Check sheet for the modelled part. Datum: model origin and axes. Units: mm. Face numbers are marked on the shaded views. A direction names the side the tool comes from. Give positions to 0.01 mm unless a question says otherwise; leave off trailing zeros. Order: outer loops, then holes, each group sorted by start corner. A loop starts at its lowest first (then second) coordinate and runs counter-clockwise, first axis right, second up.
from build123d import *

# Parameters (mm, degrees)
SKETCH1_R               = 5
BOSS_EXTRUDE1_DEPTH     = 40
SKETCH2_R               = 9
BOSS_EXTRUDE2_DEPTH     = 10
SKETCH3_R               = 5
BOSS_EXTRUDE3_DEPTH     = 10
BOSS_EXTRUDE4_DEPTH     = 20
SKETCH6_R               = 5
BOSS_EXTRUDE5_DEPTH     = 8
SKETCH5_W               = 30
SKETCH5_H               = 5.5
CUT_EXTRUDE1_DEPTH      = 10
CUT_EXTRUDE1_DEPTH_BACK = 10
SKETCH8_R               = 1.5
CUT_EXTRUDE2_DEPTH      = 2


with BuildPart() as part:
    # Sketch1 → Boss-Extrude1 (new body)
    with BuildSketch(Plane.XY):
        Circle(SKETCH1_R)
    extrude(amount=BOSS_EXTRUDE1_DEPTH)

    # Sketch2 → Boss-Extrude2 (add)
    with BuildSketch(Plane(origin=(0, 0, 0), x_dir=(-1, 0, 0), z_dir=(0, 0, -1))):
        Circle(SKETCH2_R)
    extrude(amount=BOSS_EXTRUDE2_DEPTH)

    # Sketch3 → Boss-Extrude3 (add)
    with BuildSketch(Plane(origin=(0, 0, -10), x_dir=(-1, 0, 0), z_dir=(0, 0, -1))):
        Circle(SKETCH3_R)
    extrude(amount=BOSS_EXTRUDE3_DEPTH)

    # Sketch4 → Boss-Extrude4 (add)
    with BuildSketch(Plane(origin=(0, 0, -20), x_dir=(-1, 0, 0), z_dir=(0, 0, -1))):
        Polygon((-5, 0), (-2.5, -4.330127019), (2.5, -4.330127019), (5, 0), (2.5, 4.330127019), (-2.5, 4.330127019), align=None)
    extrude(amount=BOSS_EXTRUDE4_DEPTH)

    # Sketch6 → Boss-Extrude5 (add)
    with BuildSketch(Plane.XY.offset(40)):
        Circle(SKETCH6_R)
    extrude(amount=BOSS_EXTRUDE5_DEPTH)

    # Sketch5 → Cut-Extrude1 (cut, two sides)
    with BuildSketch(Plane(origin=(0, 0, 0), x_dir=(0, 0, -1), z_dir=(1, 0, 0))) as cut_extrude1_sk:
        with Locations((-30, 2.25)):
            Rectangle(SKETCH5_W, SKETCH5_H)
    extrude(amount=CUT_EXTRUDE1_DEPTH, mode=Mode.SUBTRACT)
    extrude(cut_extrude1_sk.sketch, amount=-CUT_EXTRUDE1_DEPTH_BACK, mode=Mode.SUBTRACT)

    # Sketch8 → Cut-Extrude2 (cut)
    with BuildSketch(Plane(origin=(0, -0.5, 0), x_dir=(1, 0, 0), z_dir=(0, 1, 0))):
        with Locations((0, -40)):
            Circle(SKETCH8_R)
        with Locations((0, -20)):
            Circle(SKETCH8_R)
    extrude(amount=-CUT_EXTRUDE2_DEPTH, mode=Mode.SUBTRACT)


solid = part.part
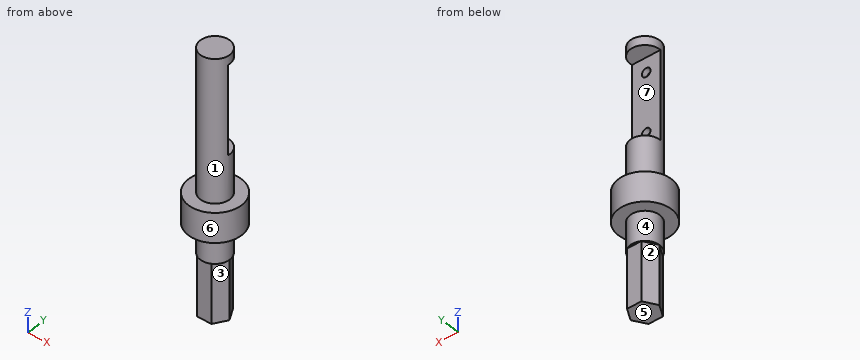
1) Draft check along Z on the marked faces 5, 6 and 7. Enter one of: +Z half, -Z half, draft (parallel to the pull), parting line (faces both ways), or undercut.
Recorded:
face 5: -Z half
face 6: draft
face 7: undercut
2) Set-up check for the marked faces 1, 2, 3 and 4: record each of +Z, -Z, +X, -X, +Y, -Y from which the full face is reachable in a straight line by a thin tool's end or side.
Recorded:
face 1: +Z
face 2: -Z, -X, +Y
face 3: -Z, +X, -Y
face 4: -Z
3) Section check B-B, the plane y = 2.25. Record the cut outline in (x, z), then the cut area to 3 significant figures.
Recorded:
outline: (-8.71, -10) - (-4.47, -10) - (-4.47, -20) - (-3.7, -20) - (-3.7, -40) - (3.7, -40) - (3.7, -20) - (4.47, -20) - (4.47, -10) - (8.71, -10) - (8.71, 0) - (4.47, 0) - (4.47, 15) - (-4.47, 15) - (-4.47, 0) - (-8.71, 0) - close; (-4.47, 45) - (4.47, 45) - (4.47, 48) - (-4.47, 48) - close
area: 572 mm2
4) Section check A-A, the plane x = 0. Record the cut outline in (y, z), then the cut area to 3 significant figures.
Recorded:
outline: (-9, -10) - (-5, -10) - (-5, -20) - (-4.33, -20) - (-4.33, -40) - (4.33, -40) - (4.33, -20) - (5, -20) - (5, -10) - (9, -10) - (9, 0) - (5, 0) - (5, 15) - (-0.5, 15) - (-0.5, 18.5) - (-2.5, 18.5) - (-2.5, 21.5) - (-0.5, 21.5) - (-0.5, 38.5) - (-2.5, 38.5) - (-2.5, 41.5) - (-0.5, 41.5) - (-0.5, 45) - (5, 45) - (5, 48) - (-5, 48) - (-5, 0) - (-9, 0) - close
area: 756 mm2
5) Section check C-C, the plane z = -28.5. Record the cut outline in (x, y).
Recorded:
outline: (-5, 0) - (-2.5, -4.33) - (2.5, -4.33) - (5, 0) - (2.5, 4.33) - (-2.5, 4.33) - close
6) Depth check by flat-ended pin: pin 1 Ø3.5 at (x, z) = (0.5, 20.5) entering from +Y; pin 2 Ø10 at (y, z) = (1.5, 21.5) entering from +X; pin 3 Ø6 at (y, z) = (-7, -30) entering from +X. Enter the tip coordinate at first touch or a pass-through.
Recorded:
pin 1: stops at y = -0.5
pin 2: stops at x = 4.97
pin 3: stops at x = 2.69
7) Material ranges on L1, parallel to Z at x = 0, y = -1.8; L2, parallel to X at y = -2.5, z = 23; L3, parallel to Z at x = 5.25, y = 0.5, recorded low to high.
Recorded:
L1: z = -40 to 18.5, 21.5 to 38.5, 41.5 to 48
L2: x = -4.33 to 4.33
L3: z = -10 to 0
